```python
from build123d import *

# Parameters (mm, degrees)
SKETCH_R      = 17.25
SKETCH_R_2    = 3.5
SKETCH_R_3    = 3
PAD_DEPTH     = 2
SKETCH003_R   = 15
SKETCH003_R_2 = 13.75
PAD001_DEPTH  = 4
SKETCH005_R   = 1.5
POCKET_DEPTH  = 2.001


with BuildPart() as part:
    # Sketch → Pad (new body)
    with BuildSketch(Plane.XY):
        Circle(SKETCH_R)
        Circle(SKETCH_R_2, mode=Mode.SUBTRACT)
        with Locations((10, 0)):
            Circle(SKETCH_R_3, mode=Mode.SUBTRACT)
        with Locations((-10, 0)):
            Circle(SKETCH_R_3, mode=Mode.SUBTRACT)
    extrude(amount=PAD_DEPTH)

    # Sketch003 (on Face6 of Pad) → Pad001 (join)
    with BuildSketch(Plane.XY.offset(2)):
        Circle(SKETCH003_R)
        Circle(SKETCH003_R_2, mode=Mode.SUBTRACT)
    extrude(amount=PAD001_DEPTH)

    # Sketch005 (on Face6 of Pad) → Pocket (cut, through all)
    with BuildSketch(Plane.XY.offset(2)):
        with Locations((-3.762222, 10.336619)):
            Circle(SKETCH005_R)
        with Locations((3.762222, 10.336619)):
            Circle(SKETCH005_R)
        with Locations((-3.762222, -10.336619)):
            Circle(SKETCH005_R)
        with Locations((3.762222, -10.336619)):
            Circle(SKETCH005_R)
    extrude(amount=-POCKET_DEPTH, mode=Mode.SUBTRACT)


solid = part.part
```
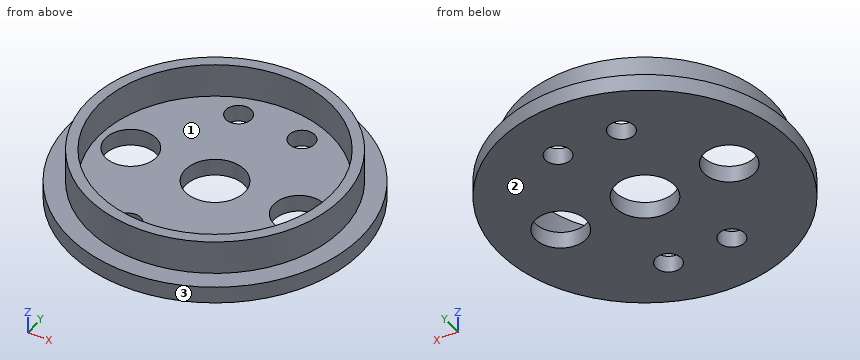
Input: part model. Units: mm. Frame: model coordinates. Face numbers are marked on the shaded views. Round coordinates to 2 decimals unless told otherwise and drop trailing zeros. Order: outer loops, then holes, each group sorted by start corner. A loop starts at its lowest first (then second) coordinate and runs counter-clockwise, first axis right, second up. Notation, with made-up numbers: (84, 63) - (141, 63) arc R22 cw to (141, 71) - close; hole circle Ø9 at (11.25, 43.25). An arc over 180 degrees is marked (long way). One line per question, with ' | ' between items. Start each with the question number.
1) Ray query, probe 1 along Y at (x, z) = (-5, 1.4); probe 2 along Z at (x, y) = (-13, -4); probe 3 along Y at (x, z) = (0, 4.9). Return the intervals inside material, ascending.
2) Cut plane B-B, the plane x = -12. Return the cut outline in (y, z), then the cut area to 3 significant figures.
3) Cut plane A-A, the plane y = 0. Return the cut outline in (x, z).
4) Cut plane C-C, the plane z = 4.15. Return the cut outline in (x, y).
5) Contact query for flat-ended pins moving along their axis: P1, Ø1, axis at x = -9, y = 6, coming from the +Z side; P2, Ø1.5, axis at x = 1.5, z = 4, coming from the -Y side. Output: stop coordinate, or through.
6) Cut plane D-D, the plane z = 1.35. Return the cut outline in (x, y), then the cut area to 3 significant figures.
7) Pull-direction query (X, two-part tool) for the marked faces 1, 2 and 3; classes: +X half, -X half, draft (parallel to the pull), parting line (faces both ways), or undercut.
Worked out:
1) probe 1: y = -16.51 to -11.18, -9.49 to 9.49, 11.18 to 16.51 | probe 2: z = 0 to 2 | probe 3: y = -15 to -13.75, 13.75 to 15
2) outline: (-12.39, 0) - (-2.24, 0) - (-2.24, 2) - (-6.71, 2) - (-6.71, 6) - (-9, 6) - (-9, 2) - (-12.39, 2) - close; (2.24, 0) - (12.39, 0) - (12.39, 2) - (9, 2) - (9, 6) - (6.71, 6) - (6.71, 2) - (2.24, 2) - close | area: 58.9 mm^2
3) outline: (-17.25, 0) - (-13, 0) - (-13, 2) - (-13.75, 2) - (-13.75, 6) - (-15, 6) - (-15, 2) - (-17.25, 2) - close; (-7, 0) - (-3.5, 0) - (-3.5, 2) - (-7, 2) - close; (3.5, 0) - (7, 0) - (7, 2) - (3.5, 2) - close; (13, 0) - (17.25, 0) - (17.25, 2) - (15, 2) - (15, 6) - (13.75, 6) - (13.75, 2) - (13, 2) - close
4) outline: circle Ø30 at (0, 0); hole circle Ø27.5 at (0, 0)
5) P1: stops at z = 2 | P2: stops at y = -14.98
6) outline: circle Ø34.5 at (0, 0); hole circle Ø6 at (-10, 0); hole circle Ø3 at (-3.76, -10.34); hole circle Ø3 at (-3.76, 10.34); hole circle Ø7 at (0, 0); hole circle Ø3 at (3.76, -10.34); hole circle Ø3 at (3.76, 10.34); hole circle Ø6 at (10, 0) | area: 812 mm^2
7) face 1: undercut | face 2: draft | face 3: parting line
